Autodesk Inventor part; units mm, degrees
ref_plane "Work Plane1" through (104.775, 0, 0) normal (0, 0, -1) x (1, 0, 0)
ref_plane "YZ Plane" through (0, 0, 0) normal (1, 0, 0) x (0, 1, 0)
ref_plane "XZ Plane" through (0, 0, 0) normal (0, 1, 0) x (-1, 0, 0)
sketch "Skizze1" plane through (0, 0, 0) normal (0, 0, 1) x (1, 0, 0)
  line L0 (8, 0) -> (8, 2)
  line L1 (8, 2) -> (5, 2)
  line L2 (5, 2) -> (4.5706, 2)
  line L3 (0, 3.765) -> (0, 1.4434)
  line L4 (0, 1.4434) -> (1.78, 1.4434)
  line L5 (1.78, 1.4434) -> (2.6133, 0)
  line L6 (2.6133, 0) -> (8, 0)
  line L7 (0, 3.765) -> (0.715, 3.765)
  line L8 (0.715, 3.765) -> (2.48, 2)
  line L9 (4.5706, 2) -> (2.48, 2)
  line L10 (5, 2) -> (2.48, 2) construction
  line L11 (2.48, 2) -> (2.48, 2)
  line L12 (-1.6, 0) -> (9.6, 0)
  line L13 (0, -0.753) -> (0, 4.518)
  dimension "d0" = 8
  dimension "d1" = 3
  dimension "d2" = 1.78
  dimension "d3" = 4
  dimension "d6" = 2.48
  dimension "d7" = 45
  dimension "d8" = 2.8868
  dimension "d9" = 60
  dimension "d10" = 7.53
  dimension "d11" = 4
  dimension "d12" = 0.4294
revolve "Körper" add sketch "Skizze1" angle 360 about axis through (2.6133, 0, 0) along (1, 0, 0) contours L6 L5 L4 L3 L7 L8 L9 L2 L1 L0
sketch "Skizze2" plane through (0, 0, 0) normal (-1, 0, 0) x (0, 0, 1)
  circle A0 centre (0, 0) radius 1.4434
  line L0 (0, -5.271) -> (0, 5.271)
  line L1 (-5.271, 0) -> (5.271, 0)
  line L2 (1.4434, 0) -> (0.7217, -1.25)
  line L3 (0.7217, -1.25) -> (-0.7217, -1.25)
  line L4 (-0.7217, -1.25) -> (-1.4434, 0)
  line L5 (-1.4434, 0) -> (-0.7217, 1.25)
  line L6 (-0.7217, 1.25) -> (0.7217, 1.25)
  line L7 (0.7217, 1.25) -> (1.4434, 0)
  point P0 (0, 1.4434)
extrude "Loch" add sketch "Skizze2" against normal up to next contours L7 A0 | A0 L2 | L6 L0 A0 | A0 L0 L3 | L0 L6 A0 | A0 L3 L0 | L4 A0 | A0 L5
thread "Gewinde"
chamfer "Fase1" distance 0.4294 distance2 0.4294 1 edges at (8, -2, 0) measured on face at (8, -0.9581, 0.5552)
ref_plane "Work Plane1" through (104.775, 0, 0) normal (0, 0, -1) x (1, 0, 0)
equation "\"d15\" = GEL"
equation "\"d17\" = -0.5 * SPD + 0.5 * GD"
equation "\"d18\" = GUL"
equation "\"d0\" = NLG"
equation "\"d1\" = GEL"
equation "\"d2\" = INTI"
equation "\"d3\" = GD"
equation "\"d6\" = KOH"
equation "\"d7\" = 0.5 * SEWI"
equation "\"d8\" = 1.1547 * SW"
equation "\"d10\" = KOD"
equation "\"d11\" = BDM"
equation "\"d12\" = GAL"
equation "\"NLG\" = 8"
equation "\"INTI\" = 1.78"
equation "\"GEL\" = 3"
equation "\"GAL\" = 0.61345 * PTC"
equation "\"KOH\" = 2.48"
equation "\"KOD\" = 7.53"
equation "\"GUL\" = 0.61345 * PTC"
equation "\"SPD\" = NND - 1.2269 * PTC"
equation "\"BDM\" = NND"
equation "\"GD\" = NND"
equation "\"SEWI\" = 90deg"
equation "\"SW\" = 2.5"
equation "\"TOA\" = 30deg"
equation "\"GD1\" = THREADDIA - 1.2269 * PTC"
equation "\"EPV\" = 4.48"
equation "\"THREADDIA\" = 4"
equation "\"PTC\" = 0.7"
equation "\"NND\" = 4"
equation "\"E0\" = 2.89"
equation "\"THREADDESC\" = 1.2345"
properties part number "ISO 10642 - M4 x  8" material "Stahl"
Geometry: final body of the model. Coordinates: model frame, mm. A direction names the side the tool comes from. Coordinates: 2 decimals unless noted, no trailing zeros. Loops run counter-clockwise (first coordinate to the right, second up) from the corner with the lowest first, then second, coordinate; pieces in that order, holes last. Notation, with made-up numbers: M 59,27 L 72,27 A16 ccw 72,44 Z; hole C -6,70 d2. An arc over 180 degrees is marked long. One line per item, written item: value. Start each with the question number.
1) Cut plane A-A (x = 6.5). Return loops of the section in (y, z).
2) Material intervals for L1, parallel to Z at x = 4.25, y = 0; L2, parallel to Z at x = 1.75, y = -0.75; L3, parallel to Z at x = 0.5, y = 2.75, sorted ascending. Write a range as from..to.
3) Draft query along Y for faces 1 (the conical face through (2.37, -0.46, 2.06)), 2 (the flat face through (8, 0, 0)), 3 (the flat face through (1, -1.25, 0)), 4 (the flat face through (0.933, -0.616, 1.088)). Return one class per face: released by +Y, released by -Y, zero draft, split by the parting line, or undercut.
4) Reachability of faces 5 (the flat face through (1, 1.25, 0)), 6 (the cylindrical face through (5, 0, 2)), 7 (the cylindrical face through (0.363, -0.49, 3.733)) from +Z, -Z, +X, -X, +Y, -Y: full face, straight path, thin tool, end or side. Return the list, or none.
5) Pin query (flat end, axial travel): P1, Ø0.7, axis at x = 1, z = -0.5, coming from the +Y side; P2, Ø3, axis at x = 5, z = -2.5, coming from the +Y side; P3, Ø3, axis at x = 4.5, z = 3, coming from the +Y side. Return the tip coordinate at first contact, or that it passes through.
Evaluation:
1. outline: C 0,0 d4
2. L1: -2..2
2. L2: -2.62..-1.01, 1.01..2.62
2. L3: -2.57..2.57
3. face 1: split by the parting line
3. face 2: zero draft
3. face 3: undercut
3. face 4: undercut
4. face 5: -X
4. face 6: +X
4. face 7: +X, -X
5. P1: y = 3.75
5. P2: y = 1.73
5. P3: y = 1.32
